Source: CAD feature listing. Evaluate the final solid. Frame: model axes, mm. A direction names the side the tool comes from. Coordinates: 2 decimals unless noted, no trailing zeros. Loops run counter-clockwise (first coordinate to the right, second up) from the corner with the lowest first, then second, coordinate; pieces in that order, holes last. Notation, with made-up numbers: (56.5, 39.5) -> (101.5, 39.5) arc R29 cw to (101.5, 59.5) -> close; hole circle Ø5 at (86, 44). An arc over 180 degrees is marked (long way). One line per question, with ' | ' between items. Start each with the question number.
```python
from build123d import *

# Parameters (mm, degrees)
F0_R     = 10
F1_DEPTH = 12
F2_DEPTH = 6
F3_DEPTH = 6


with BuildPart() as f1:
    # F0 (on Top) → F1 (new body)
    with BuildSketch(Plane.XY):
        with BuildLine():
            ThreePointArc((21.5, 0), (21.4473527551, 1.5036820799), (21.289668856, 3))
            ThreePointArc((21.289668856, 3), (15.2027957955, 15.2027957955), (3, 21.289668856))
            ThreePointArc((3, 21.289668856), (0, 21.5), (-3, 21.289668856))
            ThreePointArc((-3, 21.289668856), (-15.2027957955, 15.2027957955), (-21.289668856, 3))
            ThreePointArc((-21.289668856, 3), (-21.5, 0), (-21.289668856, -3))
            ThreePointArc((-21.289668856, -3), (-15.2027957955, -15.2027957955), (-3, -21.289668856))
            ThreePointArc((-3, -21.289668856), (0, -21.5), (3, -21.289668856))
            ThreePointArc((3, -21.289668856), (15.2027957955, -15.2027957955), (21.289668856, -3))
            ThreePointArc((21.289668856, -3), (21.4473527551, -1.5036820799), (21.5, 0))
        make_face()
        Circle(F0_R, mode=Mode.SUBTRACT)
        with BuildLine():
            Line((21.289668856, 3), (24.819347292, 3))
            ThreePointArc((24.819347292, 3), (17.6776695297, 17.6776695297), (3, 24.819347292))
            Line((3, 24.819347292), (3, 21.289668856))
            ThreePointArc((3, 21.289668856), (15.2027957955, 15.2027957955), (21.289668856, 3))
        make_face()
        with BuildLine():
            Line((3, 21.289668856), (3, 24.819347292))
            ThreePointArc((3, 24.819347292), (0, 25), (-3, 24.819347292))
            Line((-3, 24.819347292), (-3, 21.289668856))
            ThreePointArc((-3, 21.289668856), (0, 21.5), (3, 21.289668856))
        make_face()
        with BuildLine():
            Line((-3, 21.289668856), (-3, 24.819347292))
            ThreePointArc((-3, 24.819347292), (-17.6776695297, 17.6776695297), (-24.819347292, 3))
            Line((-24.819347292, 3), (-21.289668856, 3))
            ThreePointArc((-21.289668856, 3), (-15.2027957955, 15.2027957955), (-3, 21.289668856))
        make_face()
        with BuildLine():
            Line((-21.289668856, 3), (-24.819347292, 3))
            ThreePointArc((-24.819347292, 3), (-25, 0), (-24.819347292, -3))
            Line((-24.819347292, -3), (-21.289668856, -3))
            ThreePointArc((-21.289668856, -3), (-21.5, 0), (-21.289668856, 3))
        make_face()
        with BuildLine():
            ThreePointArc((-24.819347292, -3), (-17.6776695297, -17.6776695297), (-3, -24.819347292))
            Line((-3, -24.819347292), (-3, -21.289668856))
            ThreePointArc((-3, -21.289668856), (-15.2027957955, -15.2027957955), (-21.289668856, -3))
            Line((-21.289668856, -3), (-24.819347292, -3))
        make_face()
        with BuildLine():
            ThreePointArc((-3, -24.819347292), (0, -25), (3, -24.819347292))
            Line((3, -24.819347292), (3, -21.289668856))
            ThreePointArc((3, -21.289668856), (0, -21.5), (-3, -21.289668856))
            Line((-3, -21.289668856), (-3, -24.819347292))
        make_face()
        with BuildLine():
            ThreePointArc((3, -24.819347292), (17.6776695297, -17.6776695297), (24.819347292, -3))
            Line((24.819347292, -3), (21.289668856, -3))
            ThreePointArc((21.289668856, -3), (15.2027957955, -15.2027957955), (3, -21.289668856))
            Line((3, -21.289668856), (3, -24.819347292))
        make_face()
        with BuildLine():
            ThreePointArc((24.819347292, -3), (24.9547959549, -1.5027171558), (25, 0))
            ThreePointArc((25, 0), (24.9547959549, 1.5027171558), (24.819347292, 3))
            Line((24.819347292, 3), (21.289668856, 3))
            ThreePointArc((21.289668856, 3), (21.4473527551, 1.5036820799), (21.5, 0))
            ThreePointArc((21.5, 0), (21.4473527551, -1.5036820799), (21.289668856, -3))
            Line((21.289668856, -3), (24.819347292, -3))
        make_face()
    extrude(amount=F1_DEPTH)

    # F0 (on Top) → F2 (cut)
    with BuildSketch(Plane.XY):
        with BuildLine():
            ThreePointArc((21.5, 0), (21.4473527551, 1.5036820799), (21.289668856, 3))
            ThreePointArc((21.289668856, 3), (15.2027957955, 15.2027957955), (3, 21.289668856))
            ThreePointArc((3, 21.289668856), (0, 21.5), (-3, 21.289668856))
            ThreePointArc((-3, 21.289668856), (-15.2027957955, 15.2027957955), (-21.289668856, 3))
            ThreePointArc((-21.289668856, 3), (-21.5, 0), (-21.289668856, -3))
            ThreePointArc((-21.289668856, -3), (-15.2027957955, -15.2027957955), (-3, -21.289668856))
            ThreePointArc((-3, -21.289668856), (0, -21.5), (3, -21.289668856))
            ThreePointArc((3, -21.289668856), (15.2027957955, -15.2027957955), (21.289668856, -3))
            ThreePointArc((21.289668856, -3), (21.4473527551, -1.5036820799), (21.5, 0))
        make_face()
        Circle(F0_R, mode=Mode.SUBTRACT)
    extrude(amount=F2_DEPTH, mode=Mode.SUBTRACT)

    # F0 (on Top) → F3 (cut)
    with BuildSketch(Plane.XY):
        with BuildLine():
            Line((3, 21.289668856), (3, 24.819347292))
            ThreePointArc((3, 24.819347292), (0, 25), (-3, 24.819347292))
            Line((-3, 24.819347292), (-3, 21.289668856))
            ThreePointArc((-3, 21.289668856), (0, 21.5), (3, 21.289668856))
        make_face()
        with BuildLine():
            ThreePointArc((-3, -24.819347292), (0, -25), (3, -24.819347292))
            Line((3, -24.819347292), (3, -21.289668856))
            ThreePointArc((3, -21.289668856), (0, -21.5), (-3, -21.289668856))
            Line((-3, -21.289668856), (-3, -24.819347292))
        make_face()
        with BuildLine():
            Line((-21.289668856, 3), (-24.819347292, 3))
            ThreePointArc((-24.819347292, 3), (-25, 0), (-24.819347292, -3))
            Line((-24.819347292, -3), (-21.289668856, -3))
            ThreePointArc((-21.289668856, -3), (-21.5, 0), (-21.289668856, 3))
        make_face()
        with BuildLine():
            ThreePointArc((24.819347292, -3), (24.9547959549, -1.5027171558), (25, 0))
            ThreePointArc((25, 0), (24.9547959549, 1.5027171558), (24.819347292, 3))
            Line((24.819347292, 3), (21.289668856, 3))
            ThreePointArc((21.289668856, 3), (21.4473527551, 1.5036820799), (21.5, 0))
            ThreePointArc((21.5, 0), (21.4473527551, -1.5036820799), (21.289668856, -3))
            Line((21.289668856, -3), (24.819347292, -3))
        make_face()
    extrude(amount=F3_DEPTH, mode=Mode.SUBTRACT)


solid = f1.part
```
(1) Draft query along X for faces 1 (the flat face through (-16, 16, 0)), 2 (the cylindrical face through (15.065, -15.34, 2.958)). Return one class per face: pulls with the +X half, pulls with the -X half, needs draft (parallel to the pull), parting line crosses it, or undercut.
(2) Ray query, L1, parallel to Y at x = 0, z = 8.2; L2, parallel to Z at x = 4.5, y = -16; L3, parallel to Y at x = 10, z = 5.5. Return the intervals inside material, ascending.
(3) Cut plane C-C, the plane z = 8.5. Return the cut outline in (x, y).
(4) Cut plane D-D, the plane y = -8. Return the cut outline in (x, z).
(5) Cut plane B-B, the plane x = 0. Return the cut outline in (y, z).
(6) Access query for faces 3 (the flat face through (11, 0, 6)), 4 (the cylindrical face through (-2.17, -9.76, 8.96)), 5 (the flat face through (-3, 23, 3)), 6 (the flat face through (15, 16, 0)), 7 (the flat face through (-23, -3, 3)). Directions: +Z, -Z, +X, -X, +Y, -Y. A direction counts if a zero-diameter tool reaches every point of the face in a straight line with its end or side. Return the directions, or none.
(7) Contact query for flat-ended pins moving along their axis: pin 1 Ø4 at (y, z) = (-11.5, 7.5) entering from -X; pin 2 Ø3 at (y, z) = (23.5, 4) entering from -X; pin 3 Ø1.8 at (y, z) = (-22.5, 3) entering from -X; pin 4 Ø3 at (x, y) = (6.5, 4.5) entering from -Z. Output: stop coordinate, or through.
(8) Cut plane A-A, the plane z = 3.75. Return the cut outline in (x, y).
Here are the results:
1) face 1: needs draft | face 2: undercut
2) L1: y = -25 to -10, 10 to 25 | L2: z = 6 to 12 | L3: y = -22.91 to -19.03, 19.03 to 22.91
3) outline: circle Ø50 at (0, 0); hole circle Ø20 at (0, 0)
4) outline: (-23.69, 0) -> (-19.96, 0) -> (-19.96, 6) -> (-6, 6) -> (-6, 12) -> (-23.69, 12) -> close; (6, 6) -> (19.96, 6) -> (19.96, 0) -> (23.69, 0) -> (23.69, 12) -> (6, 12) -> close
5) outline: (-25, 6) -> (-10, 6) -> (-10, 12) -> (-25, 12) -> close; (10, 6) -> (25, 6) -> (25, 12) -> (10, 12) -> close
6) face 3: -Z | face 4: +Z, -Z | face 5: -Z, +Y, -Y | face 6: -Z, +X, -X, +Y, -Y | face 7: -Z, +X, -X
7) pin 1: stops at x = -23.12 | pin 2: stops at x = -11.87 | pin 3: stops at x = -12.59 | pin 4: passes through
8) outline: (-24.82, -3) arc R25 ccw to (-3, -24.82) -> (-3, -21.29) arc R21.5 cw to (-21.29, -3) -> close; (-24.82, 3) -> (-21.29, 3) arc R21.5 cw to (-3, 21.29) -> (-3, 24.82) arc R25 ccw to start; (3, -24.82) arc R25 ccw to (24.82, -3) -> (21.29, -3) arc R21.5 cw to (3, -21.29) -> close; (3, 21.29) arc R21.5 cw to (21.29, 3) -> (24.82, 3) arc R25 ccw to (3, 24.82) -> close
